Check sheet for the modelled part. Datum: model origin and axes. Units: mm. Face numbers are marked on the shaded views. A direction names the side the tool comes from. Give positions to 0.01 mm unless a question says otherwise; leave off trailing zeros. Write each loop counter-clockwise with the first axis right and the second up, starting at its lowest first coordinate (ties: lowest second). Pieces come first, ordered by that corner, then holes. Notation, with made-up numbers: (86.25, 14) -> (142.25, 14) arc R30 cw to (142.25, 49) -> close; hole circle Ø4 at (1, -29.5). An arc over 180 degrees is marked (long way). Answer as a JSON object with one key per item and string values.
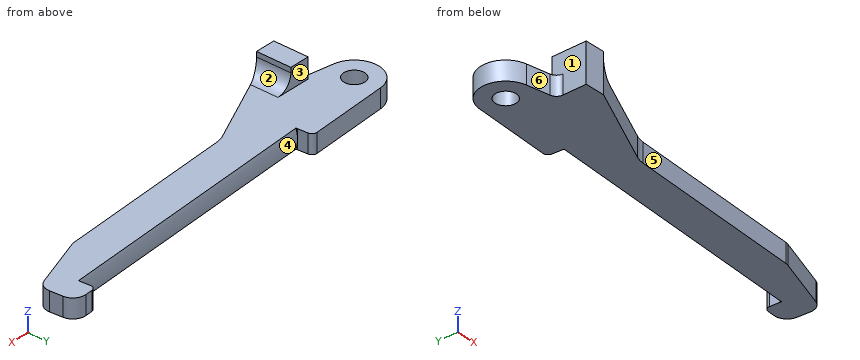
from build123d import *

# Parameters (mm, degrees)
SKETCH1_R           = 4.2
BOSS_EXTRUDE1_DEPTH = 7.6
SKETCH2_W           = 8
SKETCH2_H           = 13.917535926
BOSS_EXTRUDE2_DEPTH = 8
FILLET1_R           = 6
CUT_EXTRUDE2_DEPTH  = 110
FILLET2_R           = 2


with BuildPart() as part:
    # Sketch1 → Boss-Extrude1 (new body)
    with BuildSketch(Plane.XY):
        with BuildLine():
            Line((-1.736481777, -9.84807753), (7.520944533, -11.48041156))
            ThreePointArc((7.520944533, -11.48041156), (9.298133329, -12.50647199), (10, -14.434834819))
            Line((10, -14.434834819), (10, -23.917535926))
            Line((10, -23.917535926), (18, -23.917535926))
            Line((18, -23.917535926), (52.016628597, -8.055321506))
            ThreePointArc((52.016628597, -8.055321506), (53.739011174, -7.436922973), (55.545246477, -7.142758874))
            Line((55.545246477, -7.142758874), (127.674807922, -2.098968595))
            ThreePointArc((127.674807922, -2.098968595), (128.322865225, -2.010771867), (128.953866326, -1.838741222))
            Line((128.953866326, -1.838741222), (150.276280032, 5.503154599))
            ThreePointArc((150.276280032, 5.503154599), (152.81786837, 7.47106255), (153.636259511, 10.579529846))
            Line((153.636259511, 10.579529846), (153.276081371, 15.730317208))
            ThreePointArc((153.276081371, 15.730317208), (151.568556265, 19.15508274), (147.939478751, 20.36935509))
            Line((147.939478751, 20.36935509), (142.9516585, 20.020572722))
            Line((142.9516585, 20.020572722), (143.370197342, 14.03518842))
            Line((143.370197342, 14.03518842), (33.638151814, 6.361976308))
            Line((33.638151814, 6.361976308), (33.219612971, 12.34736061))
            Line((33.219612971, 12.34736061), (-0.697564737, 9.975640503))
            ThreePointArc((-0.697564737, 9.975640503), (-9.986295348, 0.523359562), (-1.736481777, -9.84807753))
        make_face()
        Circle(SKETCH1_R, mode=Mode.SUBTRACT)
    extrude(amount=BOSS_EXTRUDE1_DEPTH)

    # Sketch2 → Boss-Extrude2 (add)
    with BuildSketch(Plane.XY.offset(7.6)):
        with Locations((14, -16.958767963)):
            Rectangle(SKETCH2_W, SKETCH2_H)
    extrude(amount=BOSS_EXTRUDE2_DEPTH)

    # Fillet1
    fillet1_edges = [part.edges().sort_by_distance(p)[0] for p in [
        (18, -16.958767963, 7.6),
    ]]
    fillet(fillet1_edges, radius=FILLET1_R)

    # Sketch6 → Cut-Extrude2 (cut)
    with BuildSketch(Plane(origin=(22.512095066, 165.472000606, 0), x_dir=(0, 0, -1), z_dir=(-0.99756405, -0.069756474, 0))):
        with BuildLine():
            Line((-7.6, 160.116112141), (-7.6, 153.498554761))
            Line((-7.6, 153.498554761), (0, 153.498554761))
            Line((0, 153.498554761), (0, 160.116112141))
            ThreePointArc((0, 160.116112141), (-3.8, 159.498554761), (-7.6, 160.116112141))
        make_face()
    extrude(amount=-CUT_EXTRUDE2_DEPTH, mode=Mode.SUBTRACT)

    # Fillet2
    fillet2_edges = [part.edges().sort_by_distance(p)[0] for p in [
        (33.219612971, 12.34736061, 3.8),
        (142.9516585, 20.020572722, 3.8),
    ]]
    fillet(fillet2_edges, radius=FILLET2_R)


solid = part.part
1. Mould release check, pull along X, two halves, no side actions. Record for the marked faces 4, 5 and 6: released by +X, released by -X, zero draft, split by the parting line, or undercut.
Determined:
{"face 4": "undercut", "face 5": "released by +X", "face 6": "released by -X"}
2. Go/stop test with flat-tipped pins: P1, Ø21, axis at x = 66.5, y = 6, coming from the +Z side; P2, Ø2, axis at y = -19, z = 12.5, coming from the -X side; P3, Ø8, axis at x = 86, z = 10.5, coming from the +Y side. Record where each tip stops, or that it passes through.
Determined:
{"P1": "z = 7.6", "P2": "x = 10", "P3": "y = 9.76"}
3. Sectioned sample at C-C, the plane y = -17. Enter the section's corners in (x, z).
Determined:
{"outline": "(10, 0) -> (32.83, 0) -> (32.83, 7.6) -> (24, 7.6) arc R6 cw to (18, 13.6) -> (18, 15.6) -> (10, 15.6) -> close"}
4. Access from +Z, -Z, +X, -X, +Y, -Y to the whole of each face (thin tool, end or side, straight path). Record for the marked faces 1, 2 and 3.
Determined:
{"face 1": "+Z, -X, -Y", "face 2": "+Z, +X, +Y, -Y", "face 3": "+Z, +X, -X, +Y"}
5. Sectioned sample at A-A, the plane y = 0. Enter the section's corners in (x, z).
Determined:
{"outline": "(-10, 0) -> (-4.2, 0) -> (-4.2, 7.6) -> (-10, 7.6) -> close; (4.2, 0) -> (134.29, 0) -> (134.29, 7.6) -> (4.2, 7.6) -> close"}
6. Scan lines: L1, parallel to Y at x = 0, z = 4.75; L2, parallel to Z at x = 144.5, y = 15; L3, parallel to X at y = -19, z = 1.5. Record each from-to range of solid material in increasing order. Write a range as [from, to].
Determined:
{"L1": "[-10.15, -4.2], [4.2, 10.02]", "L2": "[0, 7.6]", "L3": "[10, 28.55]"}
7. Sectioned sample at B-B, the plane z = 1.75. Enter the section's corners in (x, y).
Determined:
{"outline": "(-1.74, -9.85) -> (7.52, -11.48) arc R3 cw to (10, -14.43) -> (10, -23.92) -> (18, -23.92) -> (52.02, -8.06) arc R10 cw to (55.55, -7.14) -> (127.67, -2.1) arc R5 ccw to (128.95, -1.84) -> (150.28, 5.5) arc R5 ccw to (153.64, 10.58) -> (153.28, 15.73) arc R5 ccw to (147.94, 20.37) -> (144.95, 20.16) arc R2 ccw to (143.09, 18.03) -> (143.38, 13.86) -> (33.65, 6.19) -> (33.36, 10.35) arc R2 ccw to (31.22, 12.21) -> (-0.7, 9.98) arc R10 ccw to start; hole circle Ø8.4 at (0, 0)"}
